Autodesk Inventor part; units mm, degrees
ref_plane "Work Plane1" through (-2.7515, 150, 3.6) normal (0, 1, 0) x (1, 0, 0)
ref_plane "YZ Plane" through (0, 0, 0) normal (1, 0, 0) x (0, 1, 0)
ref_plane "XZ Plane" through (0, 0, 0) normal (0, 1, 0) x (-1, 0, 0)
ref_plane "Work Plane1" through (-2.7515, 150, 3.6) normal (0, 1, 0) x (1, 0, 0)
sketch "Sketch1" plane through (-2.7515, 150, 3.6) normal (0, 1, 0) x (1, 0, 0)
  arc A0 (-6.7485, 13.6) -> (-7.2485, 13.1) centre (-6.7485, 13.1) ccw
  line L0 (-7.2485, 13.1) -> (-7.2485, 8.1)
  line L1 (-7.2485, 8.1) -> (-5.7485, 6.6)
  line L2 (-5.7485, 6.6) -> (-5.7485, 9.8)
  line L3 (-5.7485, 9.8) -> (-4.2971, 9.8)
  line L4 (-4.2971, 9.8) -> (-0.8485, 6.3515)
  line L5 (-0.8485, 6.3515) -> (-0.8485, 0.8485)
  line L6 (-0.8485, 0.8485) -> (-4.2971, -2.6)
  line L7 (-4.2971, -2.6) -> (-5.7485, -2.6)
  line L8 (-5.7485, -2.6) -> (-5.7485, 0.6)
  line L9 (-5.7485, 0.6) -> (-7.2485, -0.9)
  line L10 (-7.2485, -0.9) -> (-7.2485, -5.9)
  arc A1 (-7.2485, -5.9) -> (-6.7485, -6.4) centre (-6.7485, -5.9) ccw
  line L11 (-6.7485, -6.4) -> (-1.7485, -6.4)
  line L12 (-1.7485, -6.4) -> (-0.2485, -4.9)
  line L13 (-0.2485, -4.9) -> (-3.4485, -4.9)
  line L14 (-3.4485, -4.9) -> (-3.4485, -3.4485)
  line L15 (-3.4485, -3.4485) -> (0, 0)
  line L16 (0, 0) -> (5.5029, 0)
  line L17 (5.5029, 0) -> (8.9515, -3.4485)
  line L18 (8.9515, -3.4485) -> (8.9515, -4.9)
  line L19 (8.9515, -4.9) -> (5.7515, -4.9)
  line L20 (5.7515, -4.9) -> (7.2515, -6.4)
  line L21 (7.2515, -6.4) -> (12.2515, -6.4)
  arc A2 (12.2515, -6.4) -> (12.7515, -5.9) centre (12.2515, -5.9) ccw
  line L22 (12.7515, -5.9) -> (12.7515, -0.9)
  line L23 (12.7515, -0.9) -> (11.2515, 0.6)
  line L24 (11.2515, 0.6) -> (11.2515, -2.6)
  line L25 (11.2515, -2.6) -> (9.8, -2.6)
  line L26 (9.8, -2.6) -> (6.3515, 0.8485)
  line L27 (6.3515, 0.8485) -> (6.3515, 6.3515)
  line L28 (6.3515, 6.3515) -> (9.8, 9.8)
  line L29 (9.8, 9.8) -> (11.2515, 9.8)
  line L30 (11.2515, 9.8) -> (11.2515, 6.6)
  line L31 (11.2515, 6.6) -> (12.7515, 8.1)
  line L32 (12.7515, 8.1) -> (12.7515, 13.1)
  arc A3 (12.7515, 13.1) -> (12.2515, 13.6) centre (12.2515, 13.1) ccw
  line L33 (12.2515, 13.6) -> (7.2515, 13.6)
  line L34 (7.2515, 13.6) -> (5.7515, 12.1)
  line L35 (5.7515, 12.1) -> (8.9515, 12.1)
  line L36 (8.9515, 12.1) -> (8.9515, 10.6485)
  line L37 (8.9515, 10.6485) -> (5.5029, 7.2)
  line L38 (5.5029, 7.2) -> (0, 7.2)
  line L39 (0, 7.2) -> (-3.4485, 10.6485)
  line L40 (-3.4485, 10.6485) -> (-3.4485, 12.1)
  line L41 (-3.4485, 12.1) -> (-0.2485, 12.1)
  line L42 (-0.2485, 12.1) -> (-1.7485, 13.6)
  line L43 (-1.7485, 13.6) -> (-6.7485, 13.6)
  circle A4 centre (2.7515, 3.6) radius 2
extrude "Extrusion1" add sketch "Sketch1" along normal blind 1000
ref_plane "Work Plane2" through (0, 150, -9.5) normal (1, 0, 0) x (0, 0, -1)
ref_plane "Work Plane3" through (-4.5, 150, 0) normal (0, 0, 1) x (1, 0, 0)
ref_plane "Work Plane4" through (-2.7515, 1050, 3.6) normal (0, 1, 0) x (1, 0, 0)
ref_plane "Work Plane5" through (-2.7515, 250, 3.6) normal (0, -1, 0) x (1, 0, 0)
ref_plane "Work Plane6" through (-2.7515, 395, 3.6) normal (0, -1, 0) x (1, 0, 0)
sketch "Sketch2" plane through (-2.7515, 395, 3.6) normal (0, -1, 0) x (1, 0, 0)
  line L0 (-8.2636, 7.3901) -> (13.7161, 7.3901)
  line L1 (13.7161, 7.3901) -> (13.7161, -14.5025)
  line L2 (13.7161, -14.5025) -> (-8.2636, -14.5025)
  line L3 (-8.2636, -14.5025) -> (-8.2636, 7.3901)
  point P0 (2.7515, -3.6)
extrude "Extrusion2" cut sketch "Sketch2" against normal blind 1000
properties part number "20x20mmx150mm alminum profile" material "Aluminum 6061"
Input: part model. Units: mm. Frame: model coordinates. A direction names the side the tool comes from. Give positions to 0.01 mm unless a question says otherwise; leave off trailing zeros. Order: outer loops, then holes, each group sorted by start corner. A loop starts at its lowest first (then second) coordinate and runs counter-clockwise, first axis right, second up. Notation, with made-up numbers: M 79,69 L 136,69 A29 cw 136,98 Z; hole C 43.25,30 d10. An arc over 180 degrees is marked long. Answer as a JSON object with one key per item and string values.
1. First-contact query: P1, Ø2, axis at y = 207, z = -2.5, coming from the -X side; P2, Ø5, axis at y = 370.5, z = -1.5, coming from the +X side; P3, Ø1.5, axis at x = 1.5, y = 302.5, coming from the +Z side; P4, Ø2.5, axis at x = -4, y = 284, coming from the +Z side. Flat tips, straight axial feed; report the tip coordinate or a pass-through.
Result sheet:
{"P1": "x = -9", "P2": "x = 9.5", "P3": "z = 3.6", "P4": "z = 10"}
2. Reachability of faces 1 (the flat face through (3.6, 271, 0)), 2 (the cylindrical face through (0, 271, -2)), 3 (the flat face through (0, 271, 3.6)) from +Z, -Z, +X, -X, +Y, -Y: full face, straight path, thin tool, end or side. Return the list, or none.
Result sheet:
{"face 1": "+X, +Y, -Y", "face 2": "+Y, -Y", "face 3": "+Z, +Y, -Y"}
3. Cut plane B-B, the plane z = 0. Output: boundary loops of the cut face in (x, y), and give its area (3 significant figures).
Result sheet:
{"outline": "M -3.6,150 L -2,150 L -2,395 L -3.6,395 Z; M 2,150 L 3.6,150 L 3.6,395 L 2,395 Z", "area": "784 mm²"}
4. Ray query, line 1 (Z direction, x = 0, y = 239.5); line 2 (X direction, y = 301.5, z = 7.25). Return the intervals inside material, ascending. Write a range as [from, to].
Result sheet:
{"line 1": "[-3.6, -2], [2, 3.6]", "line 2": "[-10, -6.2], [6.2, 10]"}
5. Cut plane A-A, the plane x = 0. Output: boundary loops of the cut face in (y, z), and give its area (3 significant figures).
Result sheet:
{"outline": "M 150,-3.6 L 395,-3.6 L 395,-2 L 150,-2 Z; M 150,2 L 395,2 L 395,3.6 L 150,3.6 Z", "area": "784 mm²"}
6. Pull-direction query (X, two-part tool) for faces 4 (the flat face through (-3.6, 271, 0)), 5 (the flat face through (0, 271, -3.6)), 6 (the flat face through (10, 271, -7)), 7 (the flat face through (7, 271, -10)); classes: +X half, -X half, draft (parallel to the pull), parting line (faces both ways), or undercut.
Result sheet:
{"face 4": "-X half", "face 5": "undercut", "face 6": "+X half", "face 7": "draft"}
